Part print with two shaded views. Sizes in mm from the minimum x, y, z corner. Round coordinates to 2 decimals unless told otherwise and drop trailing zeros. Loops run counter-clockwise (first coordinate to the right, second up) from the corner with the lowest first, then second, coordinate; pieces in that order, holes last. Notation, with made-up numbers: M -4,-5.5 L 50,-5.5 A34 cw 50,28.5 Z; hole C 80,70 d1. An arc over 180 degrees is marked long. Answer as CSV lines item,"result". Start each with the question number.
Item 1: Drop flat-ended pins along their axis: pin 1 Ø1 at (x, y) = (18.5, 12.5) entering from -Z; pin 2 Ø1 at (x, y) = (31, 13) entering from +Z; pin 3 Ø1.5 at (y, z) = (2, 15.5) entering from -X. Give the stop position or say it passes through.
Item 2: Band-saw the part on A-A (z = 9). Give the cut face in (x, y), and give its area (3 significant figures).
Item 3: Wall check: line 1 (Z direction, x = 6, y = 9.5); line 2 (X direction, y = 6.25, z = 8.75); line 3 (X direction, y = 9.25, z = 6.5). Give the ranges that are in metal, low to high.
Item 4: Band-saw the part on B-B (y = 9). Give the cut face in (x, z), and give its area (3 significant figures).
Item 5: Band-saw the part on D-D (x = 65). Give the cut face in (y, z), and give its area (3 significant figures).
Item 6: Band-saw the part on C-C (x = 6). Give the cut face in (y, z).
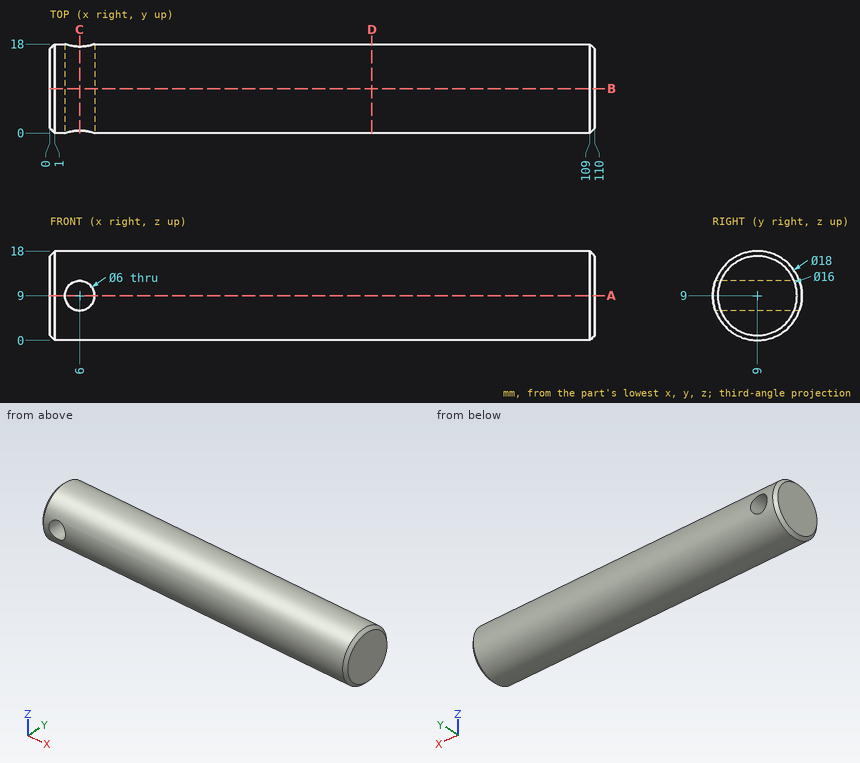
Answer block:
1,pin 1,"stops at z = 0.51"
1,pin 2,"stops at z = 17.29"
1,pin 3,"stops at x = 0.8"
2,outline,"M 0,1 L 1,0 L 3,0 L 3,18 L 1,18 L 0,17 Z; M 9,0 L 109,0 L 110,1 L 110,17 L 109,18 L 9,18 Z"
2,area,"1,870 mm^2"
3,line 1,"z = 0.01 to 6, 12 to 17.99"
3,line 2,"x = 0 to 3.01, 8.99 to 110"
3,line 3,"x = 0 to 4.34, 7.66 to 110"
4,outline,"M 0,1 L 1,0 L 109,0 L 110,1 L 110,17 L 109,18 L 1,18 L 0,17 Z; hole C 6,9 d6"
4,area,"1,950 mm^2"
5,outline,"C 9,9 d18"
5,area,"254 mm^2"
6,outline,"M 0.51,6 A9 ccw 17.49,6 Z; M 0.51,12 L 17.49,12 A9 ccw Z"
